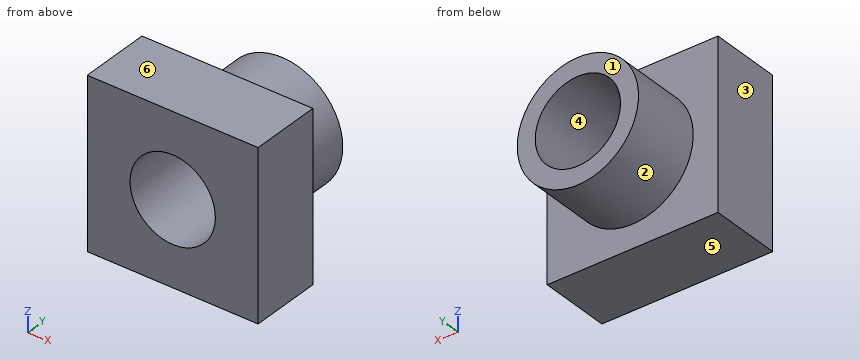
```python
from build123d import *

# Parameters (mm, degrees)
F0_W      = 60.959998
F0_H      = 59.805452
F1_DEPTH  = 25.4
F2_R      = 21.630453
F2_R_2    = 15.213086
F3_DEPTH  = 25.4
F3_FACE_R = 15.213086
F4_DEPTH  = 25.4


with BuildPart() as f1:
    # F0 (on Front) → F1 (new body)
    with BuildSketch(Plane.XZ):
        Rectangle(F0_W, F0_H)
    extrude(amount=F1_DEPTH)

    # F2 (on Front) → F3 (join, symmetric)
    with BuildSketch(Plane.XZ):
        Circle(F2_R)
        Circle(F2_R_2, mode=Mode.SUBTRACT)
    extrude(amount=F3_DEPTH, both=True)

    # F3_face (on face) → F4 (cut)
    with BuildSketch(Plane(origin=(0, 0, 0), x_dir=(1, 0, 0), z_dir=(0, 1, 0))):
        Circle(F3_FACE_R)
    extrude(amount=-F4_DEPTH, mode=Mode.SUBTRACT)


solid = f1.part
```
Work out the finished part from the listing and answer in its coordinate system (mm). Face numbers are marked on the shaded views. A direction names the side the tool comes from. Round coordinates to 2 decimals unless told otherwise and drop trailing zeros. Write each loop counter-clockwise with the first axis right and the second up, starting at its lowest first coordinate (ties: lowest second). Pieces come first, ordered by that corner, then holes.
1) Which of the six approach directions +Z, -Z, +X, -X, +Y, -Y give full straight-line access (tool end or side, diameter ignored) to the marked faces 1 and 2?
2) Flat-ended cylindrical pins translate along their axes: P1, Ø1, axis at y = 3.5, z = 2, coming from the +X side; P2, Ø5, axis at x = 7, y = 15.5, coming from the +Z side; P3, Ø6, axis at y = 16, z = -5.5, coming from the +X side. Find the tip coordinate at first contact, or state that the pin passes through.
3) A cutting plane is placed at B-B on x = 0. Determine the outline of the cut face in (y, z), and give its area (3 significant figures).
4) Determine the mould class of the marked faces 3, 4, 5 and 6 for opening direction Z: pulls with the +Z half, pulls with the -Z half, needs draft (parallel to the pull), parting line crosses it, or undercut.
5) A cutting plane is placed at A-A on z = 0. Determine the outline of the cut face in (x, y).
6) Consider probe 1 along Z at (x, y) = (0, 6); probe 2 along Y at (x, z) = (21.5, -11.5); probe 3 along Z at (x, y) = (0, -5). Determine where each line is inside the solid, lowest interval first.
7) A cutting plane is placed at C-C on y = 18. Determine the outline of the cut face in (x, z), and give its area (3 significant figures).
Entries:
1. face 1: +Z, -Z, +X, -X, +Y
1. face 2: +Y
2. P1: stops at x = 21.58
2. P2: stops at z = 21.16
2. P3: stops at x = 21.49
3. outline: (-25.4, -29.9) - (0, -29.9) - (0, -21.63) - (25.4, -21.63) - (25.4, -15.21) - (-25.4, -15.21) - close; (-25.4, 15.21) - (25.4, 15.21) - (25.4, 21.63) - (0, 21.63) - (0, 29.9) - (-25.4, 29.9) - close
3. area: 1,070 mm2
4. face 3: needs draft
4. face 4: undercut
4. face 5: pulls with the -Z half
4. face 6: pulls with the +Z half
5. outline: (-30.48, -25.4) - (-15.21, -25.4) - (-15.21, 25.4) - (-21.63, 25.4) - (-21.63, 0) - (-30.48, 0) - close; (15.21, -25.4) - (30.48, -25.4) - (30.48, 0) - (21.63, 0) - (21.63, 25.4) - (15.21, 25.4) - close
6. probe 1: z = -21.63 to -15.21, 15.21 to 21.63
6. probe 2: y = -25.4 to 0
6. probe 3: z = -29.9 to -15.21, 15.21 to 29.9
7. outline: circle Ø43.26 at (0, 0); hole circle Ø30.43 at (0, 0)
7. area: 743 mm2
